```python
from build123d import *

# Parameters (mm, degrees)
F1_DEPTH = 25
F2_R     = 10
F3_R     = 1.5
F4_DEPTH = 25
F6_DEPTH = 3


with BuildPart() as f1:
    # F0 (on Front) → F1 (new body)
    with BuildSketch(Plane.XZ):
        with BuildLine():
            ThreePointArc((-73.8, 4.65), (-46.125, 44.625), (0, 60))
            Line((0, 60), (0, 62))
            ThreePointArc((0, 62), (-47.325, 46.225), (-75.72, 5.21))
            ThreePointArc((-75.72, 5.21), (-76.6783837972, 0.7754833996), (-77, -3.75))
            Line((-77, -3.75), (-77, -14.9147645484))
            Line((-77, -14.9147645484), (-82.1204376266, -23.7836226747))
            ThreePointArc((-82.1204376266, -23.7836226747), (-83.6254711177, -28.217308368), (-83.3192426967, -32.8894512159))
            Line((-83.3192426967, -32.8894512159), (-57.1598488652, -130.5176380902))
            Line((-57.1598488652, -130.5176380902), (-55.2279972126, -130))
            Line((-55.2279972126, -130), (-81.3873910441, -32.3718131257))
            ThreePointArc((-81.3873910441, -32.3718131257), (-81.6425813949, -28.4783607525), (-80.388386819, -24.7836226747))
            Line((-80.388386819, -24.7836226747), (-75, -15.4506629333))
            Line((-75, -15.4506629333), (-75, -3.75))
            ThreePointArc((-75, -3.75), (-74.6984848098, 0.4926406871), (-73.8, 4.65))
        make_face()
        with BuildLine():
            Line((0, 62), (0, 60))
            ThreePointArc((0, 60), (46.125, 44.625), (73.8, 4.65))
            ThreePointArc((73.8, 4.65), (74.6984848098, 0.4926406871), (75, -3.75))
            Line((75, -3.75), (75, -15.4506629333))
            Line((75, -15.4506629333), (80.388386819, -24.7836226747))
            ThreePointArc((80.388386819, -24.7836226747), (81.6425813949, -28.4783607525), (81.3873910441, -32.3718131257))
            Line((81.3873910441, -32.3718131257), (55.2279972126, -130))
            Line((55.2279972126, -130), (57.1598488652, -130.5176380902))
            Line((57.1598488652, -130.5176380902), (83.3192426967, -32.8894512159))
            ThreePointArc((83.3192426967, -32.8894512159), (83.6254711177, -28.217308368), (82.1204376266, -23.7836226747))
            Line((82.1204376266, -23.7836226747), (77, -14.9147645484))
            Line((77, -14.9147645484), (77, -3.75))
            ThreePointArc((77, -3.75), (76.6783837972, 0.7754833996), (75.72, 5.21))
            ThreePointArc((75.72, 5.21), (47.325, 46.225), (0, 62))
        make_face()
    extrude(amount=F1_DEPTH)

    # F2
    f2_edges = [f1.edges().sort_by_distance(p)[0] for p in [
        (-56.193923, -25, -130.258819),
        (-56.193923, 0, -130.258819),
    ]]
    fillet(f2_edges, radius=F2_R)

    # F3 (on face) → F4 (cut)
    with BuildSketch(Plane(origin=(-49.5596666972, 0, 28.6132869086), x_dir=(0, 1, 0), z_dir=(0.8660254038, 0, -0.5))):
        with Locations((-12.5, -56.2690534246)):
            Circle(F3_R)
    extrude(amount=-F4_DEPTH, mode=Mode.SUBTRACT)

    # F5 (on face) → F6 (join)
    with BuildSketch(Plane(origin=(-84.0284228994, 0, -22.5153480572), x_dir=(0, 1, 0), z_dir=(0.9659258263, 0, 0.2588190451))):
        with BuildLine():
            Line((0, -101.2762999161), (-25, -101.2762999161))
            ThreePointArc((-25, -101.2762999161), (-22.0710678119, -108.347367728), (-15, -111.2762999161))
            Line((-15, -111.2762999161), (-10, -111.2762999161))
            ThreePointArc((-10, -111.2762999161), (-2.9289321881, -108.347367728), (0, -101.2762999161))
        make_face()
    extrude(amount=-F6_DEPTH)


solid = f1.part
```
Read the model definition and answer for the solid it produces. Units are mm, in the model's axes. A direction names the side the tool comes from. Coordinates: 2 decimals unless noted, no trailing zeros. Loops run counter-clockwise (first coordinate to the right, second up) from the corner with the lowest first, then second, coordinate; pieces in that order, holes last. Notation, with made-up numbers: (88, -15) - (133, -15) arc R19 ccw to (133, 11) - close; hole circle Ø7 at (50.5, 16). An arc over 180 degrees is marked (long way). Answer in a Markdown table with one row per item.
1. Determine the mould class of faces 1 (the face through (79.596, -12.325, -19.411)), 2 (the face through (74.69, -12.32, 0.55)), 3 (the face through (18, 0, 59)), 4 (the face through (-81.65, -12.32, -28.53)) for opening direction Z: +Z half, -Z half, draft (parallel to the pull), parting line (faces both ways), or undercut.
Conclusion:
| item | result |
|---|---|
| face 1 | +Z half |
| face 2 | undercut |
| face 3 | draft |
| face 4 | undercut |
2. Find section D-D, the plane z = 15.5. Write down the section's boundary in (x, y).
Conclusion:
| item | result |
|---|---|
| outline | (-71.92, -25) - (-69.73, -25) - (-69.73, 0) - (-71.92, 0) - close; (69.73, -25) - (71.92, -25) - (71.92, 0) - (69.73, 0) - close |
3. Given pin 1 (9 mm diameter, centred on y = -13, z = -9, fed in from +X); pin 2 (5 mm diameter, centred on y = -13, z = -3, fed in from -X); pin 3 (1.5 mm diameter, centred on x = 60, z = -105, fed in from +Y); pin 4 (1.5 mm diameter, centred on x = -50.5, y = -18, fed in from +Z), each flat-ended and moving along its own axis, determine where each tip first touches the part or whether it passes through.
Conclusion:
| item | result |
|---|---|
| pin 1 | stops at x = 77 |
| pin 2 | stops at x = -77 |
| pin 3 | passes through |
| pin 4 | stops at z = 44.33 |
4. Find section C-C, the plane x = -28.5. Write down the section's boundary in (y, z).
Conclusion:
| item | result |
|---|---|
| outline | (-25, 54.52) - (0, 54.52) - (0, 56.67) - (-25, 56.67) - close |
5. Find section A-A, the plane z = -53. Write down the section's boundary in (x, y), then the cut area to 3 significant figures.
Conclusion:
| item | result |
|---|---|
| outline | (-77.93, -25) - (-75.86, -25) - (-75.86, 0) - (-77.93, 0) - close; (75.86, -25) - (77.93, -25) - (77.93, 0) - (75.86, 0) - close |
| area | 104 mm² |
6. Straight lines are drawn through the part: line 1 (X direction, y = -4.5, z = -45); line 2 (X direction, y = -7.75, z = -66); line 3 (Z direction, x = -31.5, y = -4.5). For each, find the intervals that lie inside material, in ascending order.
Conclusion:
| item | result |
|---|---|
| line 1 | x = -80.07 to -78, 78 to 80.07 |
| line 2 | x = -74.45 to -72.38, 72.38 to 74.45 |
| line 3 | z = 53.25 to 55.44 |
7. Which of the six approach directions +Z, -Z, +X, -X, +Y, -Y give full straight-line access (tool end or side, diameter ignored) to faces 5 (the face through (70.056, -12.325, -82.387)), 6 (the face through (-57.435, -22.148, -127.478)), 7 (the face through (-75, -12, -10))?
Conclusion:
| item | result |
|---|---|
| face 5 | -Z, +X, +Y, -Y |
| face 6 | -Z, -Y |
| face 7 | +Y, -Y |
